For this review, take the finished solid that the model builds, in its own axes (mm). Face numbers are marked on the shaded views. Coordinates: 2 decimals unless noted, no trailing zeros. Write each loop counter-clockwise with the first axis right and the second up, starting at its lowest first coordinate (ties: lowest second). Pieces come first, ordered by that corner, then holes. Notation, with made-up numbers: (26.5, 13.25) -> (73.5, 13.25) arc R12 cw to (73.5, 34.25) -> close; hole circle Ø6 at (-33, 16.5). An arc over 180 degrees is marked (long way). Put each result on its own line as item: value. Start each with the question number.
Item 1: Consider section B-B on y = -6. Give the boundary of the cut face in (x, z).
Item 2: The part is to be moulded in two halves that separate along Z. For the marked faces 1, 2 and 3, say which applies: +Z half, -Z half, draft (parallel to the pull), parting line (faces both ways), or undercut.
Item 3: Consider section C-C on x = -9.5. Give the boundary of the cut face in (y, z), and give its area (3 significant figures).
Item 4: Consider section A-A on z = 20. Give the boundary of the cut face in (x, y).
Item 5: To check wall thickness, follow L1, parallel to X at y = 0.5, z = 13; L2, parallel to X at y = 10, z = 27; L3, parallel to Y at x = 17, z = 44. State the ranges of each line that lie inside material, in increasing order.
Item 6: Consider section D-D on z = 39.5. Give the boundary of the cut face in (x, y).
```python
from build123d import *

# Parameters (mm, degrees)
EXTRUDE_1_DEPTH = 48
FILLET_1_R      = 10
FILLET_3_R      = 10


with BuildPart() as part:
    # 草图1 → 凸台-拉伸1 (new body)
    with BuildSketch(Plane.XY):
        with BuildLine():
            Line((0, 20.9), (0, 25))
            Line((0, 25), (0, 48.210201589))
            Line((0, 48.210201589), (0, 50))
            Line((0, 50), (-50, 50))
            Line((-50, 50), (-50, 0))
            Line((-50, 0), (-20.9, 0))
            ThreePointArc((-20.9, 0), (-14.778531727, 14.778531727), (0, 20.9))
        make_face()
        with BuildLine():
            Line((50, 0), (20.9, 0))
            ThreePointArc((20.9, 0), (14.778531727, -14.778531727), (0, -20.9))
            Line((0, -20.9), (0, -25))
            Line((0, -25), (50, -25))
            Line((50, -25), (50, 0))
        make_face()
        with BuildLine():
            Line((50, 25), (0, 25))
            Line((0, 25), (0, 20.9))
            ThreePointArc((0, 20.9), (14.778531727, 14.778531727), (20.9, 0))
            Line((20.9, 0), (50, 0))
            Line((50, 0), (50, 25))
        make_face()
        Polygon((0, 48.210201589), (0, 25), (50, 25), (50, 50), (0, 50), align=None)
        with BuildLine():
            ThreePointArc((0, -20.9), (-14.778531727, -14.778531727), (-20.9, 0))
            Line((-20.9, 0), (-50, 0))
            Line((-50, 0), (-50, -50))
            Line((-50, -50), (50, -50))
            Line((50, -50), (50, -25))
            Line((50, -25), (0, -25))
            Line((0, -25), (0, -20.9))
        make_face()
    extrude(amount=EXTRUDE_1_DEPTH)

    # 圆角1
    fillet_1_edges = [part.edges().sort_by_distance(p)[0] for p in [
        (-50, -50, 24),
        (-50, 50, 24),
        (50, 50, 24),
        (50, -50, 24),
    ]]
    fillet(fillet_1_edges, radius=FILLET_1_R)

    # 圆角3
    fillet_3_edges = [part.edges().sort_by_distance(p)[0] for p in [
        (0, 50, 48),
        (50, 0, 48),
        (0, -50, 48),
        (-50, 0, 48),
        (-47.071067812, 47.071067812, 48),
        (-47.071067812, -47.071067812, 48),
        (47.071067812, -47.071067812, 48),
        (47.071067812, 47.071067812, 48),
    ]]
    fillet(fillet_3_edges, radius=FILLET_3_R)


solid = part.part
```
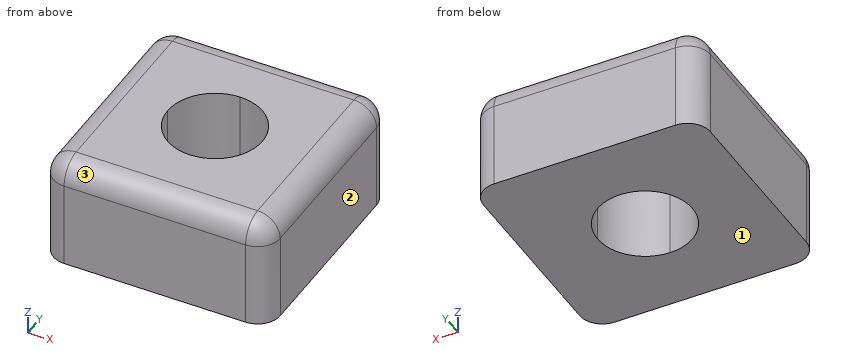
Return value:
1. outline: (-50, 0) -> (-20.02, 0) -> (-20.02, 48) -> (-40, 48) arc R10 ccw to (-50, 38) -> close; (20.02, 0) -> (50, 0) -> (50, 38) arc R10 ccw to (40, 48) -> (20.02, 48) -> close
2. face 1: -Z half
2. face 2: draft
2. face 3: +Z half
3. outline: (-50, 0) -> (-18.62, 0) -> (-18.62, 48) -> (-40, 48) arc R10 ccw to (-50, 38) -> close; (18.62, 0) -> (50, 0) -> (50, 38) arc R10 ccw to (40, 48) -> (18.62, 48) -> close
3. area: 2,970 mm^2
4. outline: (-50, -40) arc R10 ccw to (-40, -50) -> (40, -50) arc R10 ccw to (50, -40) -> (50, 40) arc R10 ccw to (40, 50) -> (-40, 50) arc R10 ccw to (-50, 40) -> close; hole circle Ø41.8 at (0, 0)
5. L1: -50 to -20.89, 20.89 to 50
5. L2: -50 to -18.35, 18.35 to 50
5. L3: -48 to -12.16, 12.16 to 48
6. outline: (-49.89, -40) arc R9.89 ccw to (-40, -49.89) -> (40, -49.89) arc R9.89 ccw to (49.89, -40) -> (49.89, 40) arc R9.89 ccw to (40, 49.89) -> (-40, 49.89) arc R9.89 ccw to (-49.89, 40) -> close; hole circle Ø41.8 at (0, 0)
